Part model, mm, in its own coordinate system. Face numbers are marked on the shaded views. A direction names the side the tool comes from. Round coordinates to 2 decimals unless told otherwise and drop trailing zeros. Write each loop counter-clockwise with the first axis right and the second up, starting at its lowest first coordinate (ties: lowest second). Pieces come first, ordered by that corner, then holes.
```python
from build123d import *

# Parameters (mm, degrees)
SKETCH1_W      = 20
SKETCH1_H      = 20
EXTRUDE1_DEPTH = 45


with BuildPart() as part:
    # Sketch1 → Extrude1 (new body)
    with BuildSketch(Plane.XY):
        Polygon((20, 0), (20, 20), (40, 20), (40, 0), (60, 0), (60, 20), (80, 20), (80, 0), (100, 0), (100, 20), (120, 20), (120, 0), (140, 0), (140, 100), (120, 100), (120, 120), (20, 120), (20, 100), (0, 100), (0, 0), align=None)
        with Locations((20, 85)):
            Rectangle(SKETCH1_W, SKETCH1_H, mode=Mode.SUBTRACT)
        with Locations((120, 85)):
            Rectangle(SKETCH1_W, SKETCH1_H, mode=Mode.SUBTRACT)
        Polygon((40, 40), (60, 40), (60, 55), (80, 55), (80, 40), (100, 40), (100, 60), (80, 60), (80, 70), (60, 70), (60, 60), (40, 60), align=None, mode=Mode.SUBTRACT)
    extrude(amount=EXTRUDE1_DEPTH)


solid = part.part
```
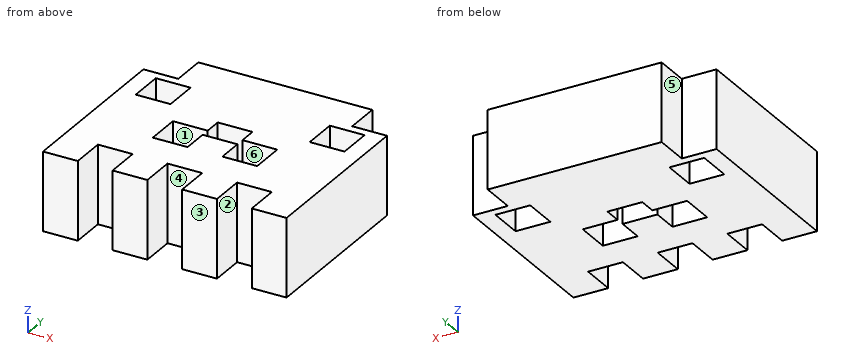
Q1. Cut at D-D on x = 15. Write the cut outline in (y, z).
Values follow:
outline: (0, 0) - (75, 0) - (75, 45) - (0, 45) - close; (95, 0) - (100, 0) - (100, 45) - (95, 45) - close
Q2. Drop flat-ended pins along their axis: pin 1 (10 mm diameter, centred on x = 27, z = 29, fed in from -Y); pin 2 (10 mm diameter, centred on x = 9.5, z = 27, fed in from +Y). Give the stop position or say it passes through.
Values follow:
pin 1: stops at y = 20
pin 2: stops at y = 100
Q3. Mould opens along Y. For the marked faces 1, 2 and 3 say: +Y half, -Y half, draft (parallel to the pull), parting line (faces both ways), or undercut.
Values follow:
face 1: undercut
face 2: draft
face 3: -Y half
Q4. Cut at C-C on y = 8.5. Write the cut outline in (x, z).
Values follow:
outline: (0, 0) - (20, 0) - (20, 45) - (0, 45) - close; (40, 0) - (60, 0) - (60, 45) - (40, 45) - close; (80, 0) - (100, 0) - (100, 45) - (80, 45) - close; (120, 0) - (140, 0) - (140, 45) - (120, 45) - close
Q5. Wall check: L1, parallel to X at y = 5.5, z = 5.5; L2, parallel to X at y = 48.5, z = 26; L3, parallel to Y at x = 13.5, z = 20. Give the ranges that are in metal, low to high.
Values follow:
L1: x = 0 to 20, 40 to 60, 80 to 100, 120 to 140
L2: x = 0 to 40, 60 to 80, 100 to 140
L3: y = 0 to 75, 95 to 100
Q6. Cut at A-A on x = 74.5. Write the cut outline in (y, z), plus the area to 4 significant figures.
Values follow:
outline: (20, 0) - (55, 0) - (55, 45) - (20, 45) - close; (70, 0) - (120, 0) - (120, 45) - (70, 45) - close
area: 3,825 mm2
Q7. Which spindle directions (+Z, -Z, +X, -X, +Y, -Y) get a long thin tool onto all of the face, cutting with end or side? Do the marked faces 4, 5 and 6. Say none if no direction does.
Values follow:
face 4: +Z, -Z, -Y
face 5: +Z, -Z, -X, +Y
face 6: +Z, -Z
Q8. Cut at B-B on y = 85. Write the cut outline in (x, z), plus the area to 3 significant figures.
Values follow:
outline: (0, 0) - (10, 0) - (10, 45) - (0, 45) - close; (30, 0) - (110, 0) - (110, 45) - (30, 45) - close; (130, 0) - (140, 0) - (140, 45) - (130, 45) - close
area: 4,500 mm2
